For this review, use the dimensioned drawing (mm, ordinates from the lowest corner) and the shaded views. Give positions to 0.01 mm unless a question says otherwise; leave off trailing zeros. Order: outer loops, then holes, each group sorted by start corner. A loop starts at its lowest first (then second) coordinate and runs counter-clockwise, first axis right, second up. Notation, with made-up numbers: M 11,71.5 L 62,71.5 A12 ccw 62,83.5 Z; hole C 61,8.25 d10. An arc over 180 degrees is marked long. Use CSV: the item, a comma, the result in double quotes. Start each with the question number.
(1) Consider section B-B (z = 10). Write out the cut boundary in (x, y), and give its area (3 significant figures).
(2) Consider section D-D (x = 22). Write out the cut boundary in (y, z) (1 decimal), and give its area (3 significant figures).
(3) Consider section C-C (y = 8.5). Write out the cut boundary in (x, z) (1 decimal).
(4) Clearance check with flat-ended pins moving along their axes: P1, Ø12, axis at x = 73, y = 22.5, coming from the +Z side; P2, Ø5, axis at x = 18, y = 11, coming from the -Z side (1 decimal); P3, Ø2, axis at x = 51.5, y = 20, coming from the -Z side. State where each tip first meets the part, or that it passes through.
(5) Wall thickness on L1, parallel to X at y = 27.5, z = 7; L2, parallel to X at y = 9.5, z = 4.5 (1 decimal); L3, parallel to Y at x = 68, z = 18.5 (1 decimal): over which ranges is each line inside the solid? List them lowest first. Write a range as from..to.
(6) Consider section A-A (y = 2). Write out the cut boundary in (x, z) (1 decimal), and give its area (3 significant figures).
(7) Draft analysis for pull direction X (two halves, no side actions). For the marked faces 1, 2 and 3, state which applies: pulls with the +X half, pulls with the -X half, needs draft (parallel to the pull), parting line crosses it, or undercut.
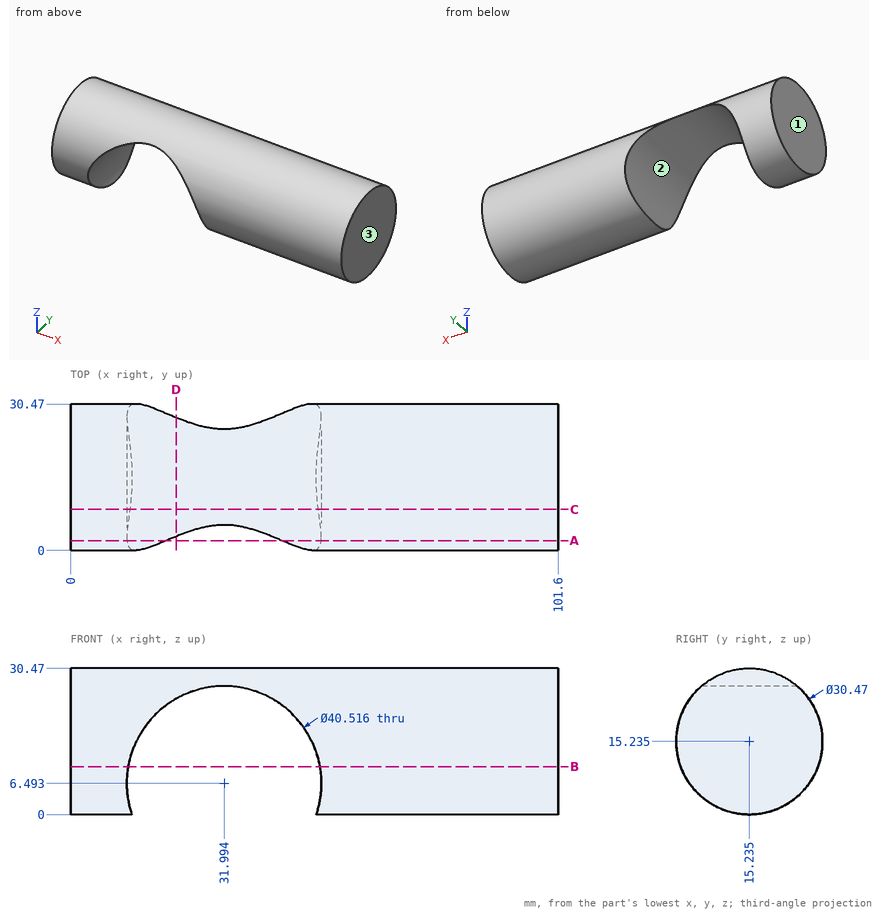
Check result:
1,outline,"M 0,0.93 L 12.04,0.93 L 12.04,29.54 L 0,29.54 Z; M 51.95,0.93 L 101.6,0.93 L 101.6,29.54 L 51.95,29.54 Z"
1,area,"1,770 mm^2"
2,outline,"M 2.9,24.1 L 27.6,24.1 A15.2 ccw Z"
2,area,"110 mm^2"
3,outline,"M 0,1.6 L 12.3,1.6 A20.3 cw long 51.6,1.6 L 101.6,1.6 L 101.6,28.9 L 0,28.9 Z"
4,P1,"stops at z = 30.42"
4,P2,"stops at z = 18.3"
4,P3,"stops at z = 0.47"
5,L1,"x = 0..11.74, 52.25..101.6"
5,L2,"x = 0..11.8, 52.2..101.6"
5,L3,"y = 0.4..30.1"
6,outline,"M 0,7.7 L 11.8,7.7 A20.3 cw 19.9,22.8 L 0,22.8 Z; M 44,22.8 A20.3 cw 52.2,7.7 L 101.6,7.7 L 101.6,22.8 Z"
6,area,"1,000 mm^2"
7,face 1,"pulls with the -X half"
7,face 2,"undercut"
7,face 3,"pulls with the +X half"
